Check sheet for the modelled part. Datum: model origin and axes. Units: mm. A direction names the side the tool comes from. Round coordinates to 2 decimals unless told otherwise and drop trailing zeros. Loops run counter-clockwise (first coordinate to the right, second up) from the corner with the lowest first, then second, coordinate; pieces in that order, holes last. Notation, with made-up numbers: M -19,78 L -9,78 A21 cw -9,107 Z; hole C 35,1 d2. An arc over 180 degrees is marked long. One line per question, with ' | ' between items. Start each with the question number.
(1) Section check A-A (z = 7.75). Record the boundary of the cut face in (x, y).
(2) Go/stop test with flat-tipped pins: P1, Ø1.5, axis at x = 102.5, z = 4, coming from the -Y side; P2, Ø9.5, axis at x = 117.5, y = 57.5, coming from the +Z side; P3, Ø4, axis at x = 47, z = 7.5, coming from the +Y side. Record where each tip stops, or that it passes through.
(3) Tool access check on faces 5 (the face through (41, 118, 7)), 6 (the face through (6, 83, 7)), 7 (the face through (118, 41, 7)). Record the directions out of +Z, -Z, +X, -X, +Y, -Y that give a thin tool (end or side, any length) a straight path to the whole face; none if there is none.
(4) Draft check along X on faces 1 (the face through (42, -5, 8)), 2 (the face through (61, 0, 4)), 3 (the face through (62, 115, 4)), 4 (the face through (112, 62, 7)). Enter one of: +X half, -X half, draft (parallel to the pull), parting line (faces both ways), or undercut.
(5) Thickness scan on probe 1 along X at (y, z) = (62, 2.65); probe 2 along Y at (x, z) = (119, 1.4). Record the ranges inside material, lowest first. Write a range as [from, to].
(6) Section check D-D (y = 62). Record the boundary of the cut face in (x, z).
(7) Section check B-B (y = 119). Record the boundary of the cut face in (x, z), and give its area (3 significant figures).
Autodesk Inventor part; units mm, degrees
ref_plane "YZ Plane" through (0, 0, 0) normal (1, 0, 0) x (0, 1, 0)
ref_plane "XZ Plane" through (0, 0, 0) normal (0, 1, 0) x (-1, 0, 0)
ref_plane "XY Plane" through (0, 0, 0) normal (0, 0, 1) x (1, 0, 0)
sketch "Sketch1" plane through (0, 0, 0) normal (0, 0, 1) x (1, 0, 0)
  line L0 (0, 0) -> (124, 0)
  line L1 (124, 0) -> (124, 124)
  line L2 (124, 124) -> (0, 124)
  line L3 (0, 124) -> (0, 0)
  circle A0 centre (5, 62) radius 2.5
  circle A1 centre (119, 62) radius 2.5
  circle A2 centre (62, 119) radius 2.5
  point P0 (124, 62)
  point P1 (0, 62)
  point P2 (62, 124)
  dimension "d0" = 124
  dimension "d1" = 124
  dimension "d2" = 5
  dimension "d3" = 5
  dimension "d4" = 5
  dimension "d5" = 5
  dimension "d6" = 5
  dimension "d7" = 5
extrude "Extrusion1" add sketch "Sketch1" along normal blind 10
sketch "Sketch2" plane through (0, 0, 10) normal (0, 0, 1) x (1, 0, 0)
  line L0 (0, 83) -> (12, 83)
  line L1 (12, 83) -> (12, 41)
  line L2 (12, 41) -> (0, 41)
  line L3 (0, 41) -> (0, 83)
  line L4 (124, 124) -> (0, 124)
  line L5 (41, 124) -> (83, 124)
  line L6 (83, 124) -> (83, 112)
  line L7 (83, 112) -> (41, 112)
  line L8 (41, 112) -> (41, 124)
  line L9 (124, 0) -> (124, 124)
  line L10 (124, 83) -> (112, 83)
  line L11 (112, 83) -> (112, 41)
  line L12 (112, 41) -> (124, 41)
  line L13 (124, 41) -> (124, 83)
  line L14 (0, 124) -> (0, 0)
  point P0 (62, 112)
  point P1 (62, 124)
  point P2 (112, 62)
  point P3 (124, 62)
  point P4 (12, 62)
  point P5 (0, 62)
  dimension "d10" = 12
  dimension "d11" = 42
  dimension "d12" = 42
  dimension "d13" = 12
  dimension "d14" = 12
  dimension "d15" = 42
extrude "Extrusion2" cut sketch "Sketch2" against normal blind 6
sketch "Sketch3" plane through (0, 0, 10) normal (0, 0, 1) x (1, 0, 0)
  line L0 (0, 0) -> (124, 0)
  line L1 (42, 0) -> (82, 0)
  line L2 (82, 0) -> (82, -10)
  line L3 (82, -10) -> (42, -10)
  line L4 (42, -10) -> (42, 0)
  circle A0 centre (62, -5) radius 2.5
  point P0 (42, -5)
  point P1 (62, -10)
  point P2 (62, 0)
  point P3 (62, 0)
  dimension "d18" = 40
  dimension "d19" = 10
  dimension "d20" = 5
extrude "Extrusion3" add sketch "Sketch3" against normal blind 5
properties part number "TC007" material "ABS Plastic"
The answers:
1) outline: M 0,0 L 42,0 L 42,-10 L 82,-10 L 82,0 L 124,0 L 124,41 L 112,41 L 112,83 L 124,83 L 124,124 L 83,124 L 83,112 L 41,112 L 41,124 L 0,124 L 0,83 L 12,83 L 12,41 L 0,41 Z; hole C 62,-5 d5
2) P1: y = 0 | P2: z = 4 | P3: y = 112
3) face 5: +Z, +Y | face 6: +Z, -X | face 7: +Z, +X
4) face 1: -X half | face 2: draft | face 3: undercut | face 4: +X half
5) probe 1: [0, 2.5], [7.5, 116.5], [121.5, 124] | probe 2: [0, 59.5], [64.5, 124]
6) outline: M 0,0 L 2.5,0 L 2.5,4 L 0,4 Z; M 7.5,0 L 116.5,0 L 116.5,4 L 112,4 L 112,10 L 12,10 L 12,4 L 7.5,4 Z; M 121.5,0 L 124,0 L 124,4 L 121.5,4 Z
7) outline: M 0,0 L 59.5,0 L 59.5,4 L 41,4 L 41,10 L 0,10 Z; M 64.5,0 L 124,0 L 124,10 L 83,10 L 83,4 L 64.5,4 Z | area: 968 mm²
